from build123d import *

# Parameters (mm, degrees)
EXTRUDE_1_DEPTH     = 10
SKETCH_2_R          = 1.5
CUT_EXTRUDE_1_DEPTH = 2
SKETCH_4_R          = 1.5
CUT_EXTRUDE_3_DEPTH = 3


with BuildPart() as part:
    # Эскиз1 → Вытянуть-Тонкостенный1 (new body)
    with BuildSketch(Plane(origin=(0, 0, 0), x_dir=(1, 0, 0), z_dir=(0, 1, 0))):
        with BuildLine():
            Line((0, 0), (-7, 0))
            ThreePointArc((-7, 0), (-21.5, -2), (-36, 0))
            Line((-36, 0), (-43, 0))
            Line((-43, 0), (-43, 2))
            Line((-43, 2), (-35.721462653, 2))
            ThreePointArc((-35.721462653, 2), (-21.5, 0), (-7.278537347, 2))
            Line((-7.278537347, 2), (0, 2))
            Line((0, 2), (0, 0))
        make_face()
    extrude(amount=EXTRUDE_1_DEPTH)

    # Эскиз2 → Вырез-Вытянуть1 (cut)
    with BuildSketch(Plane.XY):
        with Locations((-39.5, 7.5)):
            Circle(SKETCH_2_R)
        with Locations((-39.5, 2.5)):
            Circle(SKETCH_2_R)
        with Locations((-3.5, 7.5)):
            Circle(SKETCH_2_R)
        with Locations((-3.5, 2.5)):
            Circle(SKETCH_2_R)
    extrude(amount=-CUT_EXTRUDE_1_DEPTH, mode=Mode.SUBTRACT)

    # Эскиз4 → Вырез-Вытянуть3 (cut)
    with BuildSketch(Plane.XY.offset(2)):
        with Locations((-28.5, 5)):
            Circle(SKETCH_4_R)
        with Locations((-14.5, 5)):
            Circle(SKETCH_4_R)
    extrude(amount=-CUT_EXTRUDE_3_DEPTH, mode=Mode.SUBTRACT)


solid = part.part
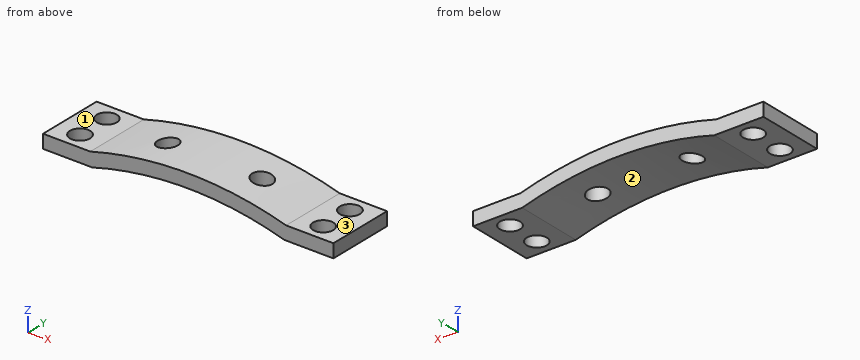
Geometry check sheet. Reference: the model listing, model coordinates, mm. Face numbers are marked on the shaded views. A direction names the side the tool comes from. Give positions to 0.01 mm unless a question says otherwise; leave off trailing zeros. Order: outer loops, then holes, each group sorted by start corner. A loop starts at its lowest first (then second) coordinate and runs counter-clockwise, first axis right, second up.
1. Scan lines: line 1 (Y direction, x = -39.5, z = -0.7); line 2 (Y direction, x = -14.5, z = 0.7); line 3 (Y direction, x = -40.5, z = -0.35). Record each from-to range of solid material in increasing order.
Completed:
line 1: y = 0 to 1, 4 to 6, 9 to 10
line 2: y = 0 to 3.5, 6.5 to 10
line 3: y = 0 to 1.38, 3.62 to 6.38, 8.62 to 10
2. Sectioned sample at B-B (x = -3.5). Record the boundary of the cut face in (y, z).
Completed:
outline: (0, -2) - (1, -2) - (1, 0) - (0, 0) - close; (4, -2) - (6, -2) - (6, 0) - (4, 0) - close; (9, -2) - (10, -2) - (10, 0) - (9, 0) - close
3. Sectioned sample at D-D (z = 0.9). Record the boundary of the cut face in (x, y), then the cut area to 3 significant figures.
Completed:
outline: (-32.3, 0) - (-10.7, 0) - (-10.7, 10) - (-32.3, 10) - close; hole circle Ø3 at (-28.5, 5); hole circle Ø3 at (-14.5, 5)
area: 202 mm2
4. Sectioned sample at A-A (y = 7.5). Record the boundary of the cut face in (x, z) (1 decimal), then the cut area to 3 significant figures.
Completed:
outline: (-43, -2) - (-41, -2) - (-41, 0) - (-43, 0) - close; (-38, -2) - (-35.7, -2) arc R51.6 cw to (-7.3, -2) - (-5, -2) - (-5, 0) - (-7, 0) arc R53.6 ccw to (-36, 0) - (-38, 0) - close; (-2, -2) - (0, -2) - (0, 0) - (-2, 0) - close
area: 74.7 mm2
5. Access from +Z, -Z, +X, -X, +Y, -Y to the whole of each face (thin tool, end or side, straight path). Record for the marked faces 1, 2 and 3.
Completed:
face 1: +Z, -X, +Y, -Y
face 2: -Z, +Y, -Y
face 3: +Z, +X, +Y, -Y
6. Sectioned sample at C-C (z = -1.35). Record the boundary of the cut face in (x, y), then the cut area to 3 significant figures.
Completed:
outline: (-43, 0) - (-33.22, 0) - (-33.22, 10) - (-43, 10) - close; (-9.78, 0) - (0, 0) - (0, 10) - (-9.78, 10) - close; hole circle Ø3 at (-39.5, 2.5); hole circle Ø3 at (-39.5, 7.5); hole circle Ø3 at (-3.5, 2.5); hole circle Ø3 at (-3.5, 7.5)
area: 167 mm2
7. Depth check by flat-ended pin: pin 1 (3.5 mm diameter, centred on x = -39.5, y = 7, fed in from +Z); pin 2 (5 mm diameter, centred on x = -24, y = 8, fed in from +Z); pin 3 (2.5 mm diameter, centred on x = -3.5, y = 7.5, fed in from +Z); pin 4 (2 mm diameter, centred on x = -34, y = 6.5, fed in from -Z). Enter the tip coordinate at first touch or a pass-through.
Completed:
pin 1: stops at z = 0
pin 2: stops at z = 2
pin 3: passes through
pin 4: stops at z = -1.8
